Verification items for this drawing (mm, ordinates from the low corner). A direction names the side the tool comes from. Coordinates: 2 decimals unless noted, no trailing zeros. Loops run counter-clockwise (first coordinate to the right, second up) from the corner with the lowest first, then second, coordinate; pieces in that order, holes last. Notation, with made-up numbers: M 78,58.25 L 83,58.25 A22 ccw 83,95.25 Z; hole C 0.5,87.25 d10. An arc over 180 degrees is marked long. Use CSV: the item, a comma, the result in double quotes.
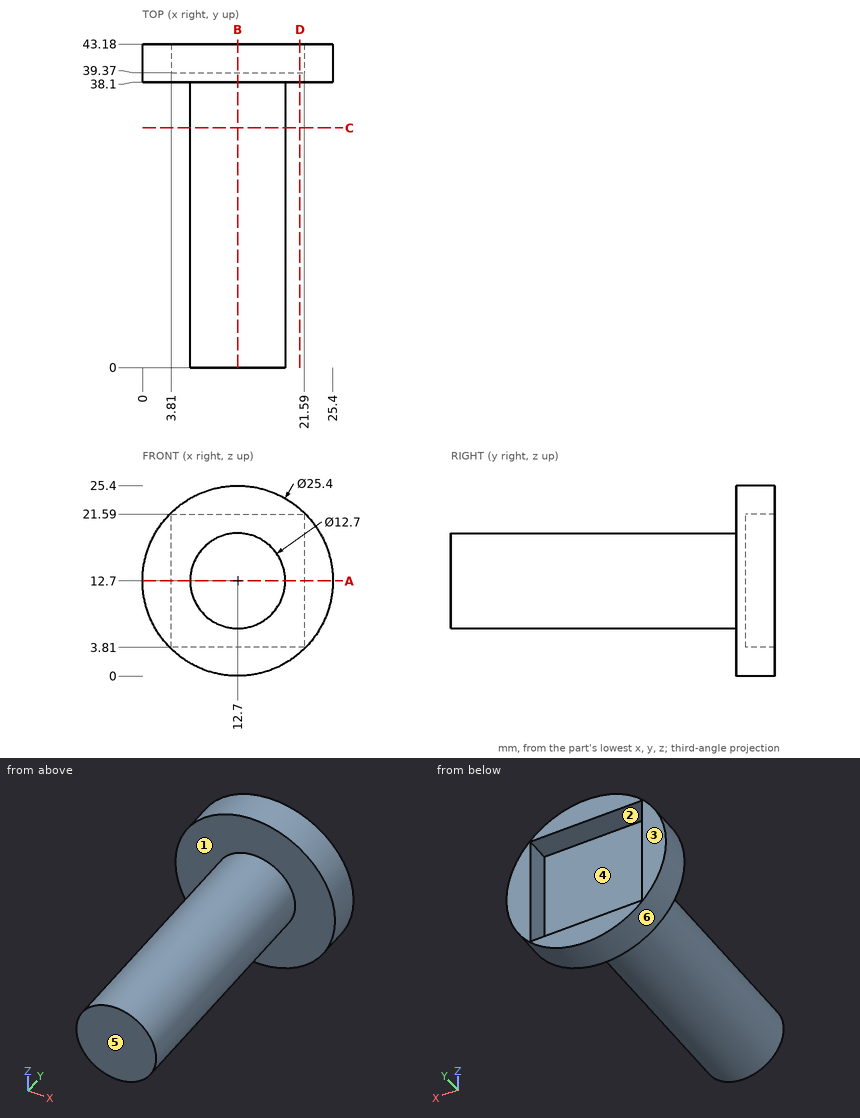
1. Section check D-D, the plane x = 21. Record the cut outline in (y, z).
The answers:
outline,"M 38.1,3.09 L 43.18,3.09 L 43.18,3.81 L 39.37,3.81 L 39.37,21.59 L 43.18,21.59 L 43.18,22.31 L 38.1,22.31 Z"
2. Section check A-A, the plane z = 12.7. Record the cut outline in (x, y), plus the area to 3 significant figures.
The answers:
outline,"M 0,38.1 L 6.35,38.1 L 6.35,0 L 19.05,0 L 19.05,38.1 L 25.4,38.1 L 25.4,43.18 L 21.59,43.18 L 21.59,39.37 L 3.81,39.37 L 3.81,43.18 L 0,43.18 Z"
area,"545 mm^2"
3. Section check C-C, the plane y = 32. Record the cut outline in (x, z).
The answers:
outline,"C 12.7,12.7 d12.7"
4. Gauge pin test, flat ends, axial feed: P1, Ø4, axis at y = 41, z = 15, coming from the +X side; P2, Ø12, axis at x = 9.5, y = 13.5, coming from the -Z side; P3, Ø3, axis at y = 12.5, z = 18, coming from the -X side. Record the tip position at first contact, or that the pin passes through.
The answers:
P1,"x = 25.4"
P2,"z = 6.35"
P3,"x = 7.61"
5. Release check for a two-part mould opening along X. For the marked faces 4, 5 and 6 record: +X half, -X half, draft (parallel to the pull), parting line (faces both ways), or undercut.
The answers:
face 4,"undercut"
face 5,"draft"
face 6,"parting line"
6. Thickness scan on line 1 (Y direction, x = 20, z = 7.75); line 2 (Y direction, x = 18.5, z = 22.5); line 3 (X direction, y = 27, z = 12.75). Record the ranges inside material, lowest first. Write a range as [from, to].
The answers:
line 1,"[38.1, 39.37]"
line 2,"[38.1, 43.18]"
line 3,"[6.35, 19.05]"
7. Section check B-B, the plane x = 12.7. Record the cut outline in (y, z).
The answers:
outline,"M 0,6.35 L 38.1,6.35 L 38.1,0 L 43.18,0 L 43.18,3.81 L 39.37,3.81 L 39.37,21.59 L 43.18,21.59 L 43.18,25.4 L 38.1,25.4 L 38.1,19.05 L 0,19.05 Z"
8. Set-up check for the marked faces 1, 2 and 3: record each of +Z, -Z, +X, -X, +Y, -Y from which the full face is reachable in a straight line by a thin tool's end or side.
The answers:
face 1,"-Y"
face 2,"+Y"
face 3,"+Z, -Z, +X, -X, +Y"
